The listing builds one solid part. Answer for the finished solid, in the listing's coordinates (mm). A direction names the side the tool comes from. Coordinates: 2 decimals unless noted, no trailing zeros. Order: outer loops, then holes, each group sorted by start corner. A loop starts at its lowest first (then second) coordinate and runs counter-clockwise, first axis right, second up. Notation, with made-up numbers: M 0.25,43.5 L 50.25,43.5 A25 ccw 50.25,75.5 Z; hole C 56.5,-30 d5. An arc over 180 degrees is marked long. One line per item, written item: value. Start each with the question number.
Q1. The part is cut by section A-A on x = 9.25. Give the vertices of the cut face in (y, z), then the cut area to 3 significant figures.
Q2. For faces 4 (the cylindrical face through (2.06, -10.72, 0.99)), 5 (the flat face through (12, 0, 2)), determine the directions among +Z, -Z, +X, -X, +Y, -Y from which every point of the face is accessible in a straight line to the end or side of a thin tool.
Q3. Determine the mould class of faces 1 (the cylindrical face through (16, 0, 1)), 2 (the cylindrical face through (2.03, 10.76, 0.99)), 3 (the flat face through (1.5, -14, 1)) for opening direction Y: pulls with the +Y half, pulls with the -Y half, needs draft (parallel to the pull), parting line crosses it, or undercut.
Q4. Straight lines are drawn through the part: line 1 along Y through (x, z) = (5.5, 0.25); line 2 along Y through (x, z) = (4.5, 0.55); line 3 along X through (y, z) = (13, 1.95). For each, find the intervals that lie inside material, in ascending order. Write a range as [from, to].
Q5. The part is cut by section D-D on y = -1. Give the vertices of the cut face in (x, z).
Q6. The part is cut by section C-C on x = 4.25. Give the vertices of the cut face in (y, z).
Q7. The part is cut by section B-B on z = 1.1. Give the vertices of the cut face in (x, y), then the cut area to 3 significant figures.
```python
from build123d import *

# Parameters (mm, degrees)
SKETCH_1_R               = 16
SKETCH_1_R_2             = 10.25
EXTRUDE_1_DEPTH          = 2
CUT_EXTRUDE_1_DEPTH      = 23.715633383
CUT_EXTRUDE_1_DEPTH_BACK = 23.715633383
FILLET_1_R               = 3


with BuildPart() as part:
    # 草图1 → 凸台-拉伸1 (new body)
    with BuildSketch(Plane.XY):
        Circle(SKETCH_1_R)
        Circle(SKETCH_1_R_2, mode=Mode.SUBTRACT)
    extrude(amount=EXTRUDE_1_DEPTH)

    # 草图2 → 切除-拉伸1 (cut, two sides: drawn at the far end of the back side and taken through both)
    with BuildSketch(Plane.XY.offset(2).offset(-CUT_EXTRUDE_1_DEPTH_BACK)):
        Polygon((1.5, 125.288041533), (1.5, 21.206511883), (1.5, -27.664442689), (1.5, -131.74597234), (-206.663059302, -131.74597234), (-206.663059302, 125.288041533), align=None)
    extrude(amount=CUT_EXTRUDE_1_DEPTH + CUT_EXTRUDE_1_DEPTH_BACK, mode=Mode.SUBTRACT)

    # 圆角1
    fillet_1_edges = [part.edges().sort_by_distance(p)[0] for p in [
        (1.5, 10.139649895, 1),
        (1.5, -10.139649895, 1),
    ]]
    fillet(fillet_1_edges, radius=FILLET_1_R)


solid = part.part
```
Output:
1. outline: M -13.06,0 L -4.42,0 L -4.42,2 L -13.06,2 Z; M 4.42,0 L 13.06,0 L 13.06,2 L 4.42,2 Z
1. area: 34.6 mm^2
2. face 4: +Z, -Z, -X
2. face 5: +Z, +X, -X, +Y, -Y
3. face 1: parting line crosses it
3. face 2: undercut
3. face 3: needs draft
4. line 1: y = [-15.02, -8.65], [8.65, 15.02]
4. line 2: y = [-15.35, -9.21], [9.21, 15.35]
4. line 3: x = [1.5, 9.33]
5. outline: M 10.2,0 L 15.97,0 L 15.97,2 L 10.2,2 Z
6. outline: M -15.43,0 L -9.33,0 L -9.33,2 L -15.43,2 Z; M 9.33,0 L 15.43,0 L 15.43,2 L 9.33,2 Z
7. outline: M 1.5,-15.93 A16 ccw 1.5,15.93 L 1.5,12.46 A3 ccw 3.48,9.64 A10.25 cw 3.48,-9.64 A3 ccw 1.5,-12.46 Z
7. area: 218 mm^2
